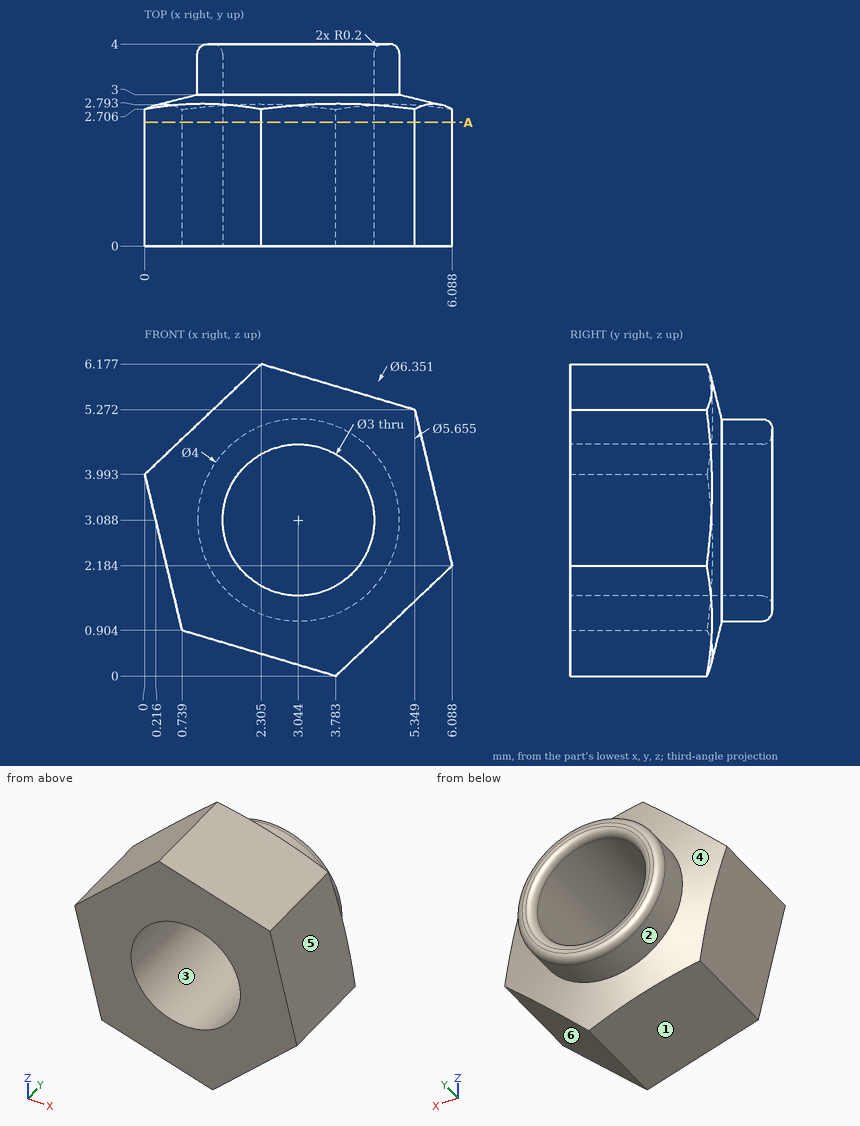
Part print with two shaded views. Sizes in mm from the minimum x, y, z corner. A direction names the side the tool comes from. Round coordinates to 2 decimals unless told otherwise and drop trailing zeros. Order: outer loops, then holes, each group sorted by start corner. A loop starts at its lowest first (then second) coordinate and runs counter-clockwise, first axis right, second up. Notation, with made-up numbers: M -19,-39.75 L 16,-39.75 A27 ccw 16,-20.75 Z; hole C 73,35.5 d11. An arc over 180 degrees is marked long. Put each result on its own line as item: value. Start each with the question number.
1. Tool access for the marked faces 1 and 2: list every direction of +Z, -Z, +X, -X, +Y, -Y with a clear straight run to the whole face (end or side of a thin tool).
2. Two-plate mould, pull along Z, no slides. Class the marked faces 3, 4, 5 and 6: +Z half, -Z half, draft (parallel to the pull), parting line (faces both ways), or undercut.
3. Drill centre lines: probe 1 along X at (y, z) = (0.6, 2.25) (1 decimal); probe 2 along X at (y, z) = (1.35, 3.5) (1 decimal); probe 3 along Z at (x, y) = (2.25, 3.55) (1 decimal). Where is each one in solid material? Low to high. Write a range as [from, to].
4. Slice it at A-A on y = 2.45. List the corners of the cut face in (x, z) (1 decimal).
5. Drop a flat-ended pin along its axis: pin 1 (2 mm diameter, centred on y = 0.5, z = 1.5, fed in from -X). Give the stop position or say it passes through.
Findings:
1. face 1: -Z, -X, +Y, -Y
1. face 2: +Y
2. face 3: undercut
2. face 4: parting line
2. face 5: +Z half
2. face 6: -Z half
3. probe 1: [0.4, 1.8], [4.3, 6.1]
3. probe 2: [0.1, 1.6], [4.5, 5.8]
3. probe 3: [1.3, 1.8], [4.4, 4.9]
4. outline: M 0,4 L 0.7,0.9 L 3.8,0 L 6.1,2.2 L 5.3,5.3 L 2.3,6.2 Z; hole C 3,3.1 d3
5. pin 1: x = 0.36
